Check sheet for the modelled part. Datum: model origin and axes. Units: mm. Face numbers are marked on the shaded views. A direction names the side the tool comes from. Round coordinates to 2 decimals unless told otherwise and drop trailing zeros. Write each loop counter-clockwise with the first axis right and the second up, starting at its lowest first coordinate (ties: lowest second). Pieces come first, ordered by that corner, then holes.
Item 1: Cross-section at C-C on z = 17. Enter the section's corners in (x, y).
Item 2: Go/stop test with flat-tipped pins: pin 1 Ø5 at (x, y) = (-1, 9) entering from +Z; pin 2 Ø1 at (y, z) = (-3.5, 20) entering from -X; pin 3 Ø1.5 at (x, y) = (0.5, 0) entering from +Z. Record where each tip stops, or that it passes through.
Item 3: Material ranges on line 1 (X direction, y = 0, z = 11); line 2 (Z direction, x = 7.5, y = 12), recorded low to high.
Item 4: Tool access check on the marked faces 1 and 2. Record the directions out of +Z, -Z, +X, -X, +Y, -Y that give a thin tool (end or side, any length) a straight path to the whole face; none if there is none.
Item 5: Cross-section at D-D on x = -10. Enter the section's corners in (y, z).
Item 6: Cross-section at A-A on y = 0. Enter the section's corners in (x, z), plus the area to 3 significant figures.
from build123d import *

# Parameters (mm, degrees)
F0_R     = 20
F1_DEPTH = 2.5
F2_R     = 3.5
F2_R_2   = 1.5
F3_DEPTH = 20
F4_R     = 5.7197863804
F4_R_2   = 3.5
F5_DEPTH = 5
F5_TAPER = 20


with BuildPart() as f1:
    # F0 (on Top) → F1 (new body)
    with BuildSketch(Plane.XY):
        Circle(F0_R)
    extrude(amount=F1_DEPTH)

    # F2 (on face) → F3 (join)
    with BuildSketch(Plane.XY.offset(2.5)):
        Circle(F2_R)
        Circle(F2_R_2, mode=Mode.SUBTRACT)
    extrude(amount=F3_DEPTH)

    # F4 (on face) → F5 (join)
    with BuildSketch(Plane.XY.offset(2.5)):
        Circle(F4_R)
        Circle(F4_R_2, mode=Mode.SUBTRACT)
        Circle(F4_R_2)
    extrude(amount=F5_DEPTH, taper=F5_TAPER)


solid = f1.part
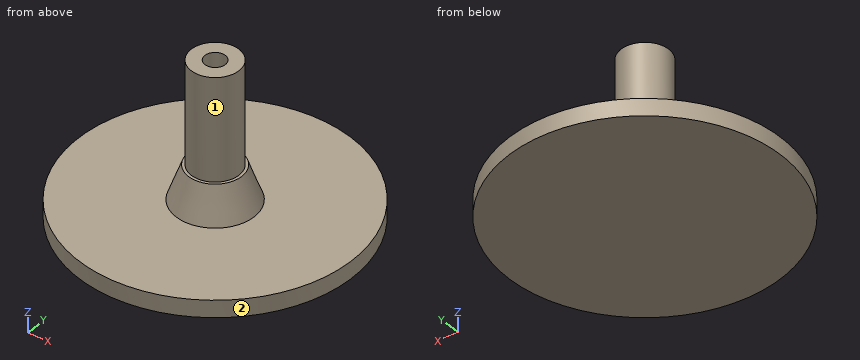
Response values:
1. outline: circle Ø7 at (0, 0); hole circle Ø3 at (0, 0)
2. pin 1: stops at z = 2.5
2. pin 2: stops at x = -1.8
2. pin 3: stops at z = 7.5
3. line 1: x = -3.5 to -1.5, 1.5 to 3.5
3. line 2: z = 0 to 2.5
4. face 1: +Z
4. face 2: +Z, -Z
5. outline: (-17.32, 0) - (17.32, 0) - (17.32, 2.5) - (-17.32, 2.5) - close
6. outline: (-20, 0) - (20, 0) - (20, 2.5) - (5.72, 2.5) - (3.9, 7.5) - (3.5, 7.5) - (3.5, 22.5) - (1.5, 22.5) - (1.5, 7.5) - (-1.5, 7.5) - (-1.5, 22.5) - (-3.5, 22.5) - (-3.5, 7.5) - (-3.9, 7.5) - (-5.72, 2.5) - (-20, 2.5) - close
6. area: 208 mm2
